```python
from build123d import *

# Parameters (mm, degrees)
F1_DEPTH = 3.29
F0_R     = 2.7
F2_DEPTH = 5.5


with BuildPart() as f1:
    # F0 (on Top) → F1 (new body)
    with BuildSketch(Plane.XY):
        with BuildLine():
            Line((18.7677565455, 12.2794405385), (6.2668947811, 13.6353748107))
            ThreePointArc((6.2668947811, 13.6353748107), (8.675985762, 12.1804513231), (9.621155417, 9.5295691997))
            ThreePointArc((9.621155417, 9.5295691997), (8.6954252879, 6.9026618527), (6.3272927871, 5.4365217026))
            Line((6.3272927871, 5.4365217026), (18.741155417, 6.7795691997))
            ThreePointArc((18.741155417, 6.7795691997), (15.9911875825, 9.5428699196), (18.7677565455, 12.2794405385))
        make_face()
        with BuildLine():
            ThreePointArc((21.491155417, 9.5295691997), (20.69508135, 11.4646850744), (18.7677565455, 12.2794405385))
            ThreePointArc((18.7677565455, 12.2794405385), (15.9911875825, 9.5428699196), (18.741155417, 6.7795691997))
            ThreePointArc((18.741155417, 6.7795691997), (20.6856990652, 7.5850255515), (21.491155417, 9.5295691997))
        make_face()
    extrude(amount=F1_DEPTH)

    # F0 (on Top) → F2 (join)
    with BuildSketch(Plane.XY):
        with BuildLine():
            Line((6.2668947811, 13.6353748107), (5.4951863181, 13.7190799162))
            ThreePointArc((5.4951863181, 13.7190799162), (1.2412777396, 9.561585585), (5.431155417, 5.3395691997))
            Line((5.431155417, 5.3395691997), (6.3272927871, 5.4365217026))
            ThreePointArc((6.3272927871, 5.4365217026), (8.6954252879, 6.9026618527), (9.621155417, 9.5295691997))
            ThreePointArc((9.621155417, 9.5295691997), (8.675985762, 12.1804513231), (6.2668947811, 13.6353748107))
        make_face()
        with Locations((5.431155417, 9.5295691997)):
            Circle(F0_R, mode=Mode.SUBTRACT)
    extrude(amount=F2_DEPTH)


solid = f1.part
```
Can you work these out from the model? Positions are in its coordinate system, mm. Give positions to 0.01 mm unless a question says otherwise; leave off trailing zeros. Order: outer loops, then holes, each group sorted by start corner. A loop starts at its lowest first (then second) coordinate and runs counter-clockwise, first axis right, second up. Notation, with made-up numbers: M -33,8.25 L 3,8.25 A25 ccw 3,47.25 Z; hole C 44,41 d7. An arc over 180 degrees is marked long. Write item = value, one per line. Start each with the question number.
Q1. Suppose I cut it at D-D (z = 2). Write out the boundary of the cut face in (x, y).
Q2. Suppose I cut it at B-B (y = 10). Write out the boundary of the cut face in (x, z), plus the area to 3 significant figures.
Q3. I need wall thicknesses on probe 1 along Z at (x, y) = (14.25, 11.75); probe 2 along X at (y, z) = (9.75, 2.5); probe 3 along X at (y, z) = (7.25, 0.65). Which ranges of each line are inside material? Lowest first, please. Write a range as [from, to].
Q4. We'd pull the mould along X, two halves only. Please class faces 1 (the flat face through (14, 10, 3.29)), 2 (the cylindrical face through (5.08, 12.207, 2.712)): pulls with the +X half, pulls with the -X half, needs draft (parallel to the pull), parting line crosses it, or undercut.
Q5. Suppose I cut it at A-A (z = 5). Write out the boundary of the cut face in (x, y), plus the area to 3 significant figures.
Q6. Will these pins go through, and if not, where does the flat tip stop? pin 1 Ø1.5 at (y, z) = (8, 2) entering from -X; pin 2 Ø2 at (x, y) = (19, 6.5) entering from -Z.
Q7. Suppose I cut it at C-C (x = 4.5). Write out the boundary of the cut face in (y, z).
Check result:
q1.outline = M 5.43,5.34 L 18.74,6.78 A2.75 ccw 18.77,12.28 L 5.5,13.72 A4.19 ccw long Z; hole C 5.43,9.53 d5.4
q2.outline = M 1.27,0 L 2.77,0 L 2.77,5.5 L 1.27,5.5 Z; M 8.09,0 L 21.45,0 L 21.45,3.29 L 9.59,3.29 L 9.59,5.5 L 8.09,5.5 Z
q2.area = 55.6 mm2
q3.probe_1 = [0, 3.29]
q3.probe_2 = [1.25, 2.74], [8.12, 21.48]
q3.probe_3 = [1.92, 3.98], [6.88, 20.28]
q4.face_1 = needs draft
q4.face_2 = undercut
q5.outline = M 5.43,5.34 L 6.33,5.44 A4.19 ccw 6.27,13.64 L 5.5,13.72 A4.19 ccw long Z; hole C 5.43,9.53 d5.4
q5.area = 32.2 mm2
q6.pin_1 = 1.31
q6.pin_2 = 0
q7.outline = M 5.44,0 L 7,0 L 7,5.5 L 5.44,5.5 Z; M 12.06,0 L 13.61,0 L 13.61,5.5 L 12.06,5.5 Z
